Autodesk Inventor part; units mm, degrees
ref_plane "YZ Plane" through (0, 0, 0) normal (1, 0, 0) x (0, 1, 0)
ref_plane "XZ Plane" through (0, 0, 0) normal (0, 1, 0) x (-1, 0, 0)
ref_plane "XY Plane" through (0, 0, 0) normal (0, 0, 1) x (1, 0, 0)
sketch "Sketch1" plane through (0, 0, 0) normal (0, 0, 1) x (1, 0, 0)
  line L0 (120, -15) -> (120, -15)
  line L1 (105, -30) -> (15, -30)
  line L2 (0, -15) -> (0, -15)
  line L3 (13.5, -10) -> (16.5, -10)
  line L4 (16.5, -10) -> (16.5, -20)
  line L5 (16.5, -20) -> (13.5, -20)
  line L6 (13.5, -20) -> (13.5, -10)
  line L7 (103.5, -10) -> (106.5, -10)
  line L8 (106.5, -10) -> (106.5, -20)
  line L9 (106.5, -20) -> (103.5, -20)
  line L10 (103.5, -20) -> (103.5, -10)
  arc A0 (15, 0) -> (0, -15) centre (15, -15) ccw
  arc A1 (0, -15) -> (15, -30) centre (15, -15) ccw
  arc A2 (105, -30) -> (120, -15) centre (105, -15) ccw
  arc A3 (120, -15) -> (105, 0) centre (105, -15) ccw
  line L11 (65, 0) -> (65, -3)
  line L12 (65, -3) -> (55, -3)
  line L13 (55, -3) -> (55, 0)
  line L14 (15, 0) -> (55, 0)
  line L15 (65, 0) -> (105, 0)
  line L16 (90, -13) -> (90, -21)
  line L17 (30, -21) -> (30, -13)
  arc A4 (35, -8) -> (30, -13) centre (35, -13) ccw
  arc A5 (90, -13) -> (85, -8) centre (85, -13) ccw
  arc A6 (85, -26) -> (90, -21) centre (85, -21) ccw
  arc A7 (30, -21) -> (35, -26) centre (35, -21) ccw
  line L18 (65, -13) -> (65, -21)
  line L19 (55, -21) -> (55, -13)
  line L20 (35, -8) -> (50, -8)
  line L21 (70, -8) -> (85, -8)
  line L22 (85, -26) -> (70, -26)
  line L23 (50, -26) -> (35, -26)
  arc A8 (55, -13) -> (50, -8) centre (50, -13) ccw
  arc A9 (50, -26) -> (55, -21) centre (50, -21) ccw
  arc A10 (65, -21) -> (70, -26) centre (70, -21) ccw
  arc A11 (70, -8) -> (65, -13) centre (70, -13) ccw
  circle A12 centre (6.868, -6.868) radius 1
  circle A13 centre (6.868, -23.132) radius 1
  circle A14 centre (23.132, -23.132) radius 1
  circle A15 centre (23.132, -6.868) radius 1
  circle A16 centre (113.132, -6.868) radius 1
  circle A17 centre (96.868, -6.868) radius 1
  circle A18 centre (96.868, -23.132) radius 1
  circle A19 centre (113.132, -23.132) radius 1
  point P0 (0, 0)
  point P1 (120, 0)
  point P2 (0, -30)
  dimension "d0" = 30
  dimension "d1" = 120
  dimension "d2" = 10
  dimension "d3" = 3
  dimension "d4" = 13.5
  dimension "d5" = 10
  dimension "d6" = 87
  dimension "d7" = 3
  dimension "d8" = 10
  dimension "d9" = 10
  dimension "d10" = 15
  dimension "d11" = 10
  dimension "d12" = 55
  dimension "d13" = 3
  dimension "d18" = 30
  dimension "d19" = 30
  dimension "d20" = 5
  dimension "d23" = 25
  dimension "d24" = 25
  dimension "d25" = 5
  dimension "d27" = 8
  dimension "d30" = 2
  dimension "d31" = 8.132
  dimension "d32" = 8.132
  dimension "d35" = 360
  dimension "d37" = 2
  dimension "d40" = 8.132
  dimension "d41" = 8.132
  dimension "d44" = 360
  dimension "d48" = 18
  dimension "d50" = 3
  dimension "d51" = 15
extrude "Extrusion4" add sketch "Sketch1" along normal blind 3
properties part number "OpenROV 2_3 Dev Horizontal Motor Mount"
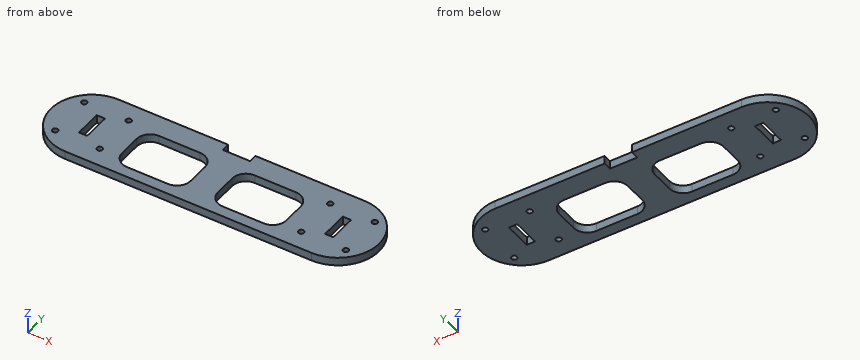
Design review of the part built by this model. Coordinates are the model's own, in mm. Coordinates: 2 decimals unless noted, no trailing zeros. Write each loop counter-clockwise with the first axis right and the second up, starting at its lowest first coordinate (ties: lowest second). Pieces come first, ordered by that corner, then holes. Notation, with made-up numbers: (33.25, 19) - (92.25, 19) arc R23 cw to (92.25, 44) - close; hole circle Ø4 at (77.25, -23.5). An arc over 180 degrees is marked (long way). One line per item, written item: value.
1) Add section A-A (y = -15). State the section outline as (x, z) points.
Answer sheet:
outline: (0, 0) - (13.5, 0) - (13.5, 3) - (0, 3) - close; (16.5, 0) - (30, 0) - (30, 3) - (16.5, 3) - close; (55, 0) - (65, 0) - (65, 3) - (55, 3) - close; (90, 0) - (103.5, 0) - (103.5, 3) - (90, 3) - close; (106.5, 0) - (120, 0) - (120, 3) - (106.5, 3) - close
2) Insertion check: pin 1 (0.9 mm diameter, centred on y = -17, z = 1.5, fed in from -X); pin 2 (3 mm diameter, centred on x = 96, y = -12.5, fed in from -Z); pin 3 (1.5 mm diameter, centred on y = -2, z = 1.5, fed in from -X); pin 4 (1.6 mm diameter, centred on x = 96.868, y = -6.868, fed in from -Z). Each pin has a flat end and moves straight along its axis. Give the tip position at first contact, or say it passes through.
Answer sheet:
pin 1: stops at x = 0.08
pin 2: stops at z = 0
pin 3: stops at x = 6.34
pin 4: passes through
3) Add section B-B (z = 2.5). Give the number of separate pieces and of enclosed holes in the cut face, plus the area to 3 significant figures.
Answer sheet:
separate pieces: 1
enclosed holes: 12
area: 2,430 mm2
4) To check wall thickness, follow probe 1 along X at (y, z) = (-12.75, 2.1); probe 2 along X at (y, z) = (-24.75, 1.7); probe 3 along X at (y, z) = (-25.25, 0.7). State the ranges of each line that lie inside material, in increasing order.
Answer sheet:
probe 1: x = 0.17 to 13.5, 16.5 to 30.01, 54.99 to 65.01, 89.99 to 103.5, 106.5 to 119.83
probe 2: x = 3.6 to 31.69, 53.31 to 66.69, 88.31 to 116.4
probe 3: x = 4.05 to 32.37, 52.63 to 67.37, 87.63 to 115.95
5) Add section C-C (y = -27.5). State the section outline as (x, z) points.
Answer sheet:
outline: (6.71, 0) - (113.29, 0) - (113.29, 3) - (6.71, 3) - close
